Here's the drawing with two shaded views (mm, measured from the low corner). I have some questions. A direction names the side the tool comes from. Coordinates: 2 decimals unless noted, no trailing zeros. Write each loop counter-clockwise with the first axis right and the second up, starting at its lowest first coordinate (ties: lowest second). Pieces come first, ordered by that corner, then holes. Notation, with made-up numbers: (22, -2.75) -> (50, -2.75) arc R18 cw to (50, 18.25) -> close; hole circle Ø9 at (-32, -18). An arc over 180 degrees is marked (long way). Use one line per item in the form item = value.
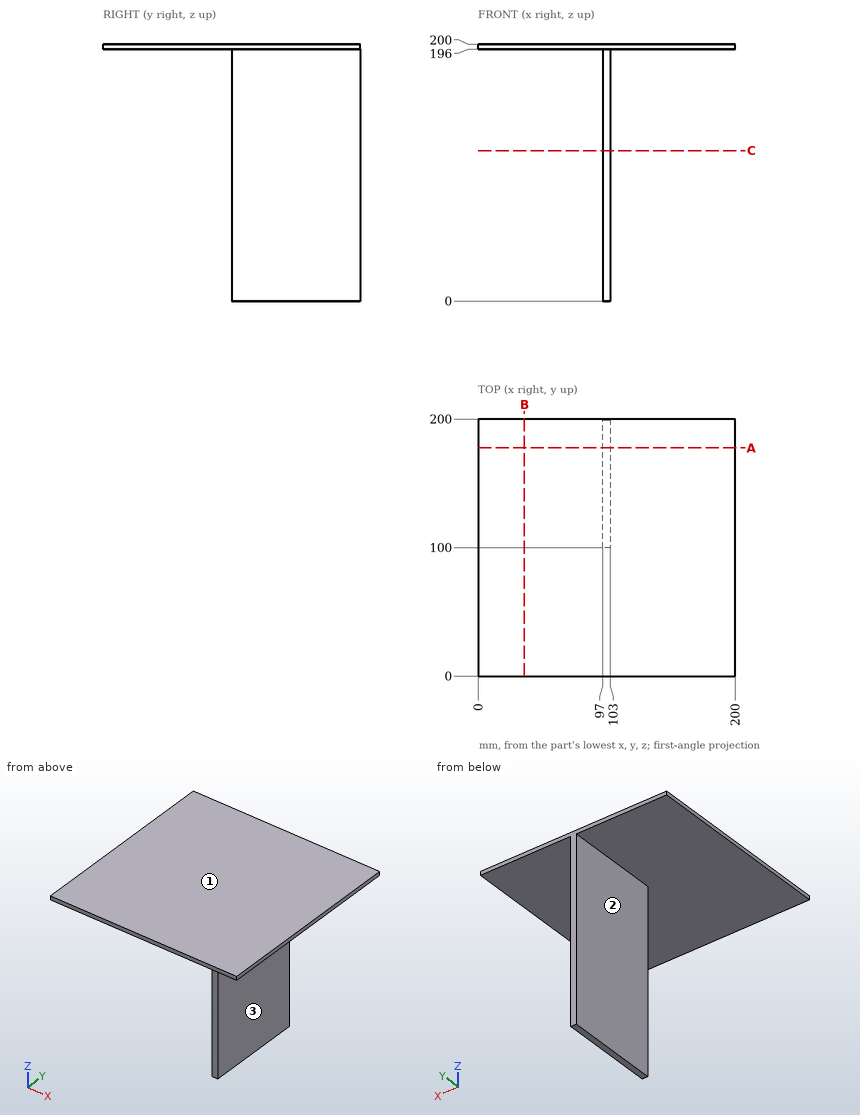
Q1. Suppose I cut it at A-A (y = 177.5). Write out the boundary of the cut face in (x, z).
Return value:
outline = (0, 196) -> (97, 196) -> (97, 0) -> (103, 0) -> (103, 196) -> (200, 196) -> (200, 200) -> (0, 200) -> close
Q2. Will these pins go through, and if not, where does the flat tip stop? pin 1 (5 mm diameter, centred on x = 98.5, z = 74.5, fed in from -Y); pin 2 (12 mm diameter, centred on x = 176.5, y = 138.5, fed in from -Z); pin 3 (8 mm diameter, centred on y = 119, z = 139, fed in from +X).
Return value:
pin_1 = 100
pin_2 = 196
pin_3 = 103
Q3. If I drill on line 1 (Z direction, x = 178, y = 133.5); line 2 (X direction, y = 173, z = 75.5), over which ranges is the centre line in solid material (lowest first)? Write a range as from..to.
Return value:
line_1 = 196..200
line_2 = 97..103
Q4. Suppose I cut it at C-C (z = 117). Write out the boundary of the cut face in (x, y).
Return value:
outline = (97, 100) -> (103, 100) -> (103, 200) -> (97, 200) -> close
Q5. Suppose I cut it at B-B (x = 36). Write out the boundary of the cut face in (y, z).
Return value:
outline = (0, 196) -> (200, 196) -> (200, 200) -> (0, 200) -> close
Q6. For the marked faces 1, 2 and 3, which set-ups out of +Z, -Z, +X, -X, +Y, -Y let a thin tool reach every point of the face, with its end or its side?
Return value:
face_1 = +Z, +X, -X, +Y, -Y
face_2 = -Z, -X, +Y, -Y
face_3 = -Z, +X, +Y, -Y
